Answer from the drawing. Dimensions are ordinates in mm from the lowest x, y and z of the part. A direction names the side the tool comes from. Coordinates: 2 decimals unless noted, no trailing zeros. Write each loop counter-clockwise with the first axis right and the second up, starting at its lowest first coordinate (ties: lowest second). Pieces come first, ordered by that corner, then holes. Notation, with made-up numbers: (46, 39) - (84, 39) arc R30 cw to (84, 62) - close; hole circle Ø10 at (56, 42). An arc over 180 degrees is marked (long way). Return JSON: item names as keys, results as strings.
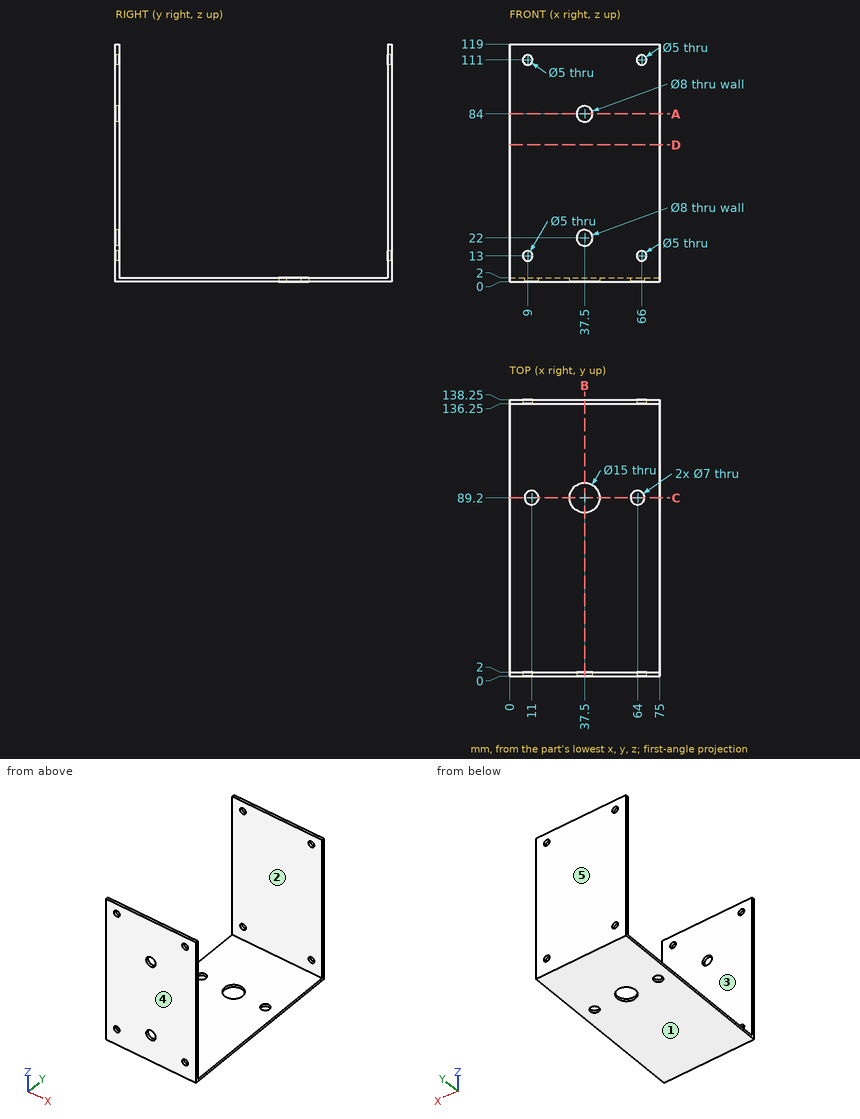
(1) A cutting plane is placed at B-B (x = 37.5). Determine the outline of the cut face in (y, z).
Answer:
{"outline": "(0, 0) - (81.7, 0) - (81.7, 2) - (2, 2) - (2, 18) - (0, 18) - close; (0, 26) - (2, 26) - (2, 80) - (0, 80) - close; (0, 88) - (2, 88) - (2, 119) - (0, 119) - close; (96.7, 0) - (138.25, 0) - (138.25, 119) - (136.25, 119) - (136.25, 2) - (96.7, 2) - close"}
(2) Determine the mould class of the marked faces 3, 4 and 5 for opening direction Y: +Y half, -Y half, draft (parallel to the pull), parting line (faces both ways), or undercut.
Answer:
{"face 3": "undercut", "face 4": "-Y half", "face 5": "+Y half"}
(3) Straight lines are drawn through the part: line 1 (X direction, y = 1.5, z = 111); line 2 (Y direction, x = 19.5, z = 36); line 3 (Z direction, x = 9, y = 137.75). For each, find the intervals that lie inside material, in ascending order. Write a range as from..to.
Answer:
{"line 1": "0..6.5, 11.5..63.5, 68.5..75", "line 2": "0..2, 136.25..138.25", "line 3": "0..10.5, 15.5..108.5, 113.5..119"}
(4) A cutting plane is placed at A-A (z = 84). Determine the outline of the cut face in (x, y).
Answer:
{"outline": "(0, 0) - (33.5, 0) - (33.5, 2) - (0, 2) - close; (0, 136.25) - (75, 136.25) - (75, 138.25) - (0, 138.25) - close; (41.5, 0) - (75, 0) - (75, 2) - (41.5, 2) - close"}
(5) Flat-ended cylindrical pins translate along their axes: P1, Ø9, axis at x = 64, y = 89.2, coming from the +Z side; P2, Ø19.5, axis at x = 37.5, y = 89.2, coming from the -Z side; P3, Ø3, axis at x = 66, z = 13, coming from the -Y side; P4, Ø7, axis at x = 37.5, z = 84, coming from the -Y side. Find the tip coordinate at first contact, or state that the pin passes through.
Answer:
{"P1": "z = 2", "P2": "z = 0", "P3": "through", "P4": "y = 136.25"}
(6) A cutting plane is placed at D-D (z = 68.5). Determine the outline of the cut face in (x, y).
Answer:
{"outline": "(0, 0) - (75, 0) - (75, 2) - (0, 2) - close; (0, 136.25) - (75, 136.25) - (75, 138.25) - (0, 138.25) - close"}
(7) Which of the six approach directions +Z, -Z, +X, -X, +Y, -Y give full straight-line access (tool end or side, diameter ignored) to the marked faces 1 and 2?
Answer:
{"face 1": "-Z, +X, -X, +Y, -Y", "face 2": "+Z, +X, -X"}
(8) A cutting plane is placed at C-C (y = 89.2). Determine the outline of the cut face in (x, z).
Answer:
{"outline": "(0, 0) - (7.5, 0) - (7.5, 2) - (0, 2) - close; (14.5, 0) - (30, 0) - (30, 2) - (14.5, 2) - close; (45, 0) - (60.5, 0) - (60.5, 2) - (45, 2) - close; (67.5, 0) - (75, 0) - (75, 2) - (67.5, 2) - close"}
